Source: CAD feature listing. Evaluate the final solid. Frame: model axes, mm. A direction names the side the tool comes from. Give positions to 0.01 mm unless a question says otherwise; leave off trailing zeros. Order: outer loops, then holes, each group sorted by start corner. A loop starts at its lowest first (then second) coordinate and runs counter-clockwise, first axis right, second up. Notation, with made-up numbers: (16, 15) -> (21, 15) arc R23 ccw to (21, 50) -> close; hole circle Ø6 at (10.25, 82.5). An arc over 180 degrees is marked (long way). Answer in a Markdown table with one row per item.
```python
from build123d import *

# Parameters (mm, degrees)
SKETCH056_W             = 28.8
SKETCH056_H             = 5
PAD024_DEPTH            = 1
SKETCH057_W             = 16
SKETCH057_H             = 2
PAD025_DEPTH            = 2
SKETCH058_R             = 0.8
POCKET026_DEPTH         = 5
CHAMFER023_SIZE         = 0.2
BODY019_PLACEMENT_ANGLE = 180


with BuildPart() as part:
    # Sketch056 → Pad024 (new body)
    with BuildSketch(Plane.YZ):
        with Locations((0, 7.7)):
            Rectangle(SKETCH056_W, SKETCH056_H)
    extrude(amount=-PAD024_DEPTH)

    # Sketch057 → Pad025 (join)
    with BuildSketch(Plane.YZ):
        with Locations((0, 7.7)):
            Rectangle(SKETCH057_W, SKETCH057_H)
    extrude(amount=-PAD025_DEPTH)

    # Sketch058 → Pocket026 (cut)
    with BuildSketch(Plane.YZ):
        with Locations((-13, 7.7)):
            Circle(SKETCH058_R)
        with Locations((13, 7.7)):
            Circle(SKETCH058_R)
    extrude(amount=-POCKET026_DEPTH, mode=Mode.SUBTRACT)

    # Chamfer023
    chamfer023_edges = [part.edges().sort_by_distance(p)[0] for p in [
        (0, -13.8, 7.7),
        (0, 12.2, 7.7),
    ]]
    chamfer(chamfer023_edges, length=CHAMFER023_SIZE)


with BuildPart() as part_1:
    # Body019 placement: moved
    add(part.part.moved(Location((25.8, 0, -0.5))).rotate(Axis((25.8, 0, -0.5), (0, 0, 1)), BODY019_PLACEMENT_ANGLE))


solid = part_1.part
```
(1) Ray query, probe 1 along Z at (x, y) = (26.5, -13); probe 2 along Y at (x, z) = (26.25, 6.6); probe 3 along Y at (x, z) = (26.5, 7.55). Return the intervals inside material, ascending.
A:
| item | result |
|---|---|
| probe 1 | z = 4.7 to 6.4, 8 to 9.7 |
| probe 2 | y = -14.4 to -13.53, -12.47 to 12.47, 13.53 to 14.4 |
| probe 3 | y = -14.4 to -13.72, -12.28 to 12.28, 13.72 to 14.4 |
(2) Section query D-D (x = 26.55). Return the cut outline in (y, z).
A:
| item | result |
|---|---|
| outline | (-14.4, 4.7) -> (14.4, 4.7) -> (14.4, 9.7) -> (-14.4, 9.7) -> close; hole circle Ø1.6 at (-13, 7.2); hole circle Ø1.6 at (13, 7.2) |
(3) Pull-direction query (Y, two-part tool) for faces 1 (the cylindrical face through (26.394, -12.896, 7.993)), 2 (the flat face through (27, -8, 7)), 3 (the flat face through (26, 0, 4.7)), 4 (the cylindrical face through (26.394, 13.104, 7.993)); classes: +Y half, -Y half, draft (parallel to the pull), parting line (faces both ways), or undercut.
A:
| item | result |
|---|---|
| face 1 | undercut |
| face 2 | -Y half |
| face 3 | draft |
| face 4 | undercut |
(4) First-contact query: pin 1 Ø0.5 at (x, z) = (27.5, 7) entering from +Y; pin 2 Ø1.8 at (y, z) = (-13, 7.2) entering from +X; pin 3 Ø1 at (y, z) = (-8, 6) entering from +X; pin 4 Ø1.4 at (y, z) = (13, 7.2) entering from +X. Flat tips, straight axial feed; report the tip coordinate or a pass-through.
A:
| item | result |
|---|---|
| pin 1 | stops at y = 8 |
| pin 2 | stops at x = 26.8 |
| pin 3 | stops at x = 27.8 |
| pin 4 | passes through |
(5) Section query C-C (y = -0.75). Return the cut outline in (x, z).
A:
| item | result |
|---|---|
| outline | (25.8, 4.7) -> (26.8, 4.7) -> (26.8, 6.2) -> (27.8, 6.2) -> (27.8, 8.2) -> (26.8, 8.2) -> (26.8, 9.7) -> (25.8, 9.7) -> close |
(6) Section query B-B (y = -13). Return the cut outline in (x, z).
A:
| item | result |
|---|---|
| outline | (25.8, 4.7) -> (26.8, 4.7) -> (26.8, 6.4) -> (26, 6.4) -> (25.8, 6.2) -> close; (25.8, 8.2) -> (26, 8) -> (26.8, 8) -> (26.8, 9.7) -> (25.8, 9.7) -> close |
(7) Section query A-A (z = 7.2). Return the cut outline in (x, y).
A:
| item | result |
|---|---|
| outline | (25.8, -14.4) -> (26.8, -14.4) -> (26.8, -13.8) -> (26, -13.8) -> (25.8, -14) -> close; (25.8, -12) -> (26, -12.2) -> (26.8, -12.2) -> (26.8, -8) -> (27.8, -8) -> (27.8, 8) -> (26.8, 8) -> (26.8, 12.2) -> (26, 12.2) -> (25.8, 12) -> close; (25.8, 14) -> (26, 13.8) -> (26.8, 13.8) -> (26.8, 14.4) -> (25.8, 14.4) -> close |
(8) Access query for faces 5 (the flat face through (27, 0, 6.2)), 6 (the flat face through (27, 0, 8.2)), 7 (the flat face through (26, 0, 9.7)), 8 (the flat face through (27, 8, 7)), 9 (the flat face through (25.8, 0, 7)). Directions: +Z, -Z, +X, -X, +Y, -Y. A direction counts if a zero-diameter tool reaches every point of the face in a straight line with its end or side. Return the directions, or none.
A:
| item | result |
|---|---|
| face 5 | -Z, +X, +Y, -Y |
| face 6 | +Z, +X, +Y, -Y |
| face 7 | +Z, +X, -X, +Y, -Y |
| face 8 | +Z, -Z, +X, +Y |
| face 9 | +Z, -Z, -X, +Y, -Y |
